Build history of the part. All positions in model axes, mm. Round coordinates to 2 decimals unless told otherwise and drop trailing zeros. Write each loop counter-clockwise with the first axis right and the second up, starting at its lowest first coordinate (ties: lowest second). Pieces come first, ordered by that corner, then holes.
from build123d import *

# Parameters (mm, degrees)
SKETCH_R   = 5
SKETCH_R_2 = 2
PAD_DEPTH  = 1
FILLET_R   = 5


with BuildPart() as part:
    # Sketch → Pad (new body)
    with BuildSketch(Plane.XY):
        Polygon((0, 0), (275, 0), (325, 42.5), (410, 42.5), (410, 82.5), (325, 82.5), (275, 125), (0, 125), align=None)
        with Locations((395, 62.5)):
            Circle(SKETCH_R, mode=Mode.SUBTRACT)
        with Locations((258.5, 116.25)):
            Circle(SKETCH_R_2, mode=Mode.SUBTRACT)
        with Locations((158.9, 8.75)):
            Circle(SKETCH_R_2, mode=Mode.SUBTRACT)
        with Locations((16.5, 116.25)):
            Circle(SKETCH_R_2, mode=Mode.SUBTRACT)
    extrude(amount=PAD_DEPTH)

    # Fillet
    fillet_edges = [part.edges().sort_by_distance(p)[0] for p in [
        (0, 0, 0.5),
        (275, 0, 0.5),
        (325, 42.5, 0.5),
        (410, 42.5, 0.5),
        (410, 82.5, 0.5),
        (325, 82.5, 0.5),
        (275, 125, 0.5),
        (0, 125, 0.5),
    ]]
    fillet(fillet_edges, radius=FILLET_R)


solid = part.part
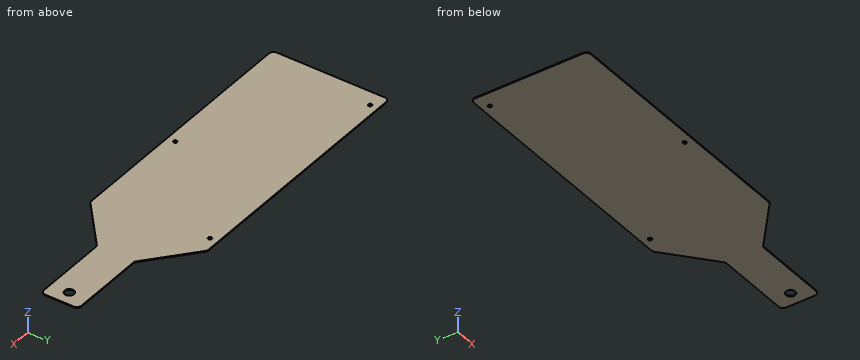
1) Slice it at C-C (y = 102.5). Write the cut outline in (x, z), plus the area to 3 significant figures.
Results:
outline: (0, 0) - (301.47, 0) - (301.47, 1) - (0, 1) - close
area: 301 mm2
2) Pin check, flat tip, straight feed: pin 1 Ø0.5 at (x, z) = (379.5, 0.5) entering from +Y. Stop position of the tip, or through.
Results:
pin 1: stops at y = 82.5
3) Slice it at B-B (z = 0.85). Write the cut outline in (x, y).
Results:
outline: (0, 5) arc R5 ccw to (5, 0) - (273.16, 0) arc R5 ccw to (276.4, 1.19) - (323.6, 41.31) arc R5 cw to (326.84, 42.5) - (405, 42.5) arc R5 ccw to (410, 47.5) - (410, 77.5) arc R5 ccw to (405, 82.5) - (326.84, 82.5) arc R5 cw to (323.6, 83.69) - (276.4, 123.81) arc R5 ccw to (273.16, 125) - (5, 125) arc R5 ccw to (0, 120) - close; hole circle Ø4 at (16.5, 116.25); hole circle Ø4 at (158.9, 8.75); hole circle Ø4 at (258.5, 116.25); hole circle Ø10 at (395, 62.5)
4) Slice it at D-D (x = 299.5). Write the cut outline in (y, z) (3 decimals), plus the area to 4 significant figures.
Results:
outline: (20.825, 0) - (104.175, 0) - (104.175, 1) - (20.825, 1) - close
area: 83.35 mm2
5) Wall check: L1, parallel to Y at x = 258.5, z = 0.35; L2, parallel to X at y = 114.5, z = 0.1; L3, parallel to X at y = 118, z = 0.75. Give the ranges that are in metal, low to high.
Results:
L1: y = 0 to 114.25, 118.25 to 125
L2: x = 0 to 15.53, 17.47 to 257.53, 259.47 to 287.35
L3: x = 0 to 15.53, 17.47 to 257.53, 259.47 to 283.24
6) Slice it at A-A (x = 395). Write the cut outline in (y, z), plus the area to 3 significant figures.
Results:
outline: (42.5, 0) - (57.5, 0) - (57.5, 1) - (42.5, 1) - close; (67.5, 0) - (82.5, 0) - (82.5, 1) - (67.5, 1) - close
area: 30.0 mm2
